Job drawing, mm, ordinate dimensions from the low corner. One solid piece. Give positions to 0.01 mm unless a question says otherwise; leave off trailing zeros. Order: outer loops, then holes, each group sorted by start corner. A loop starts at its lowest first (then second) coordinate and runs counter-clockwise, first axis right, second up. Notation, with made-up numbers: (-29.75, 52) -> (-10.75, 52) arc R10 cw to (-10.75, 58) -> close; hole circle Ø2 at (22.25, 22). An arc over 180 degrees is marked (long way). Use CSV: the item, a comma, the result in double quotes. Start each with the question number.
1. Cut at D-D on x = 15. List the corners of the cut face in (y, z).
2. Wall check: line 1 (Z direction, x = 1, y = 7.5); line 2 (Y direction, x = 2.1, z = 37); line 3 (Y direction, x = 12.75, z = 23). Give the ranges that are in metal, low to high. Write a range as from..to.
3. Cut at C-C on y = 33. List the corners of the cut face in (x, z).
4. Cut at A-A on x = 10. List the corners of the cut face in (y, z), then the cut area to 3 significant figures.
5. Cut at B-B on z = 32.5. List the corners of the cut face in (x, y), then the cut area to 3 significant figures.
6. Drop flat-ended pins along their axis: pin 1 (12 mm diameter, centred on x = 4, z = 36.5, fed in from -Y); pin 2 (5 mm diameter, centred on x = 2, z = 39, fed in from +Y); pin 3 (2 mm diameter, centred on y = 7.5, z = 37, fed in from -X). Give the stop position or say it passes through.
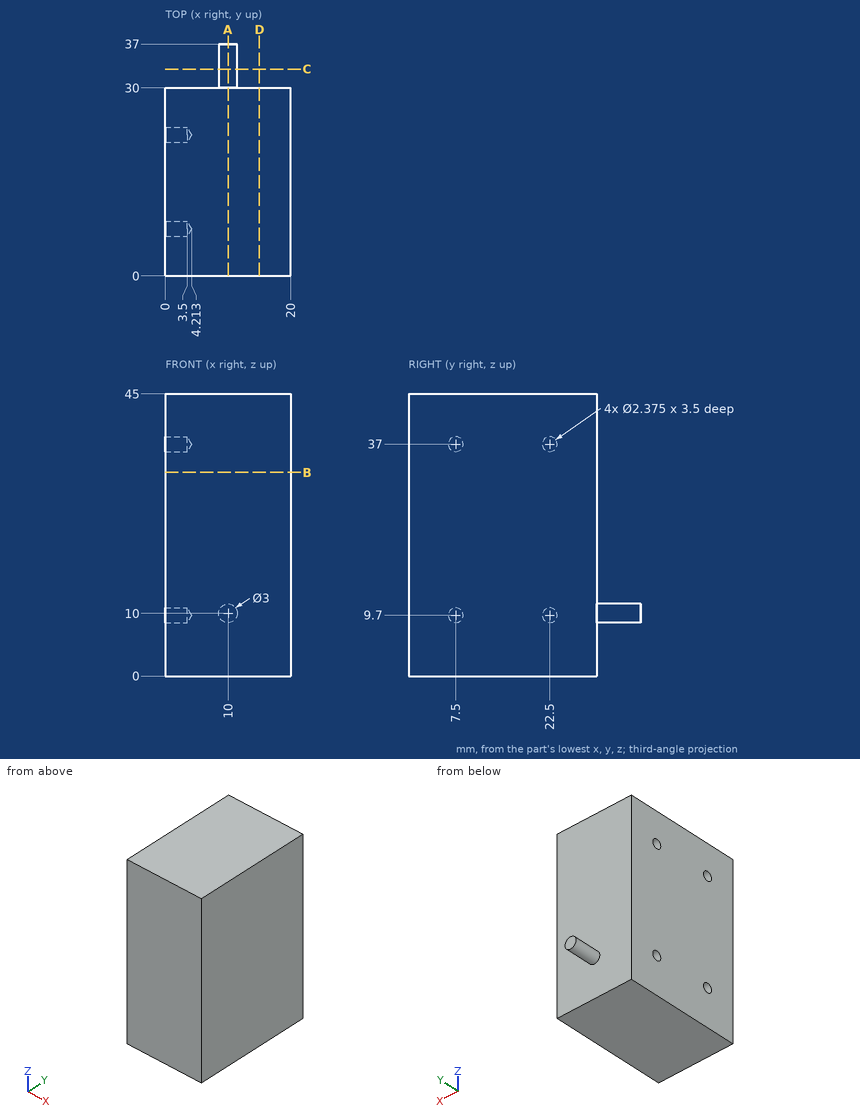
Verdict:
1,outline,"(0, 0) -> (30, 0) -> (30, 45) -> (0, 45) -> close"
2,line 1,"0..8.51, 10.89..35.81, 38.19..45"
2,line 2,"0..6.31, 8.69..21.31, 23.69..30"
2,line 3,"0..30"
3,outline,"circle Ø3 at (10, 10)"
4,outline,"(0, 0) -> (30, 0) -> (30, 8.5) -> (37, 8.5) -> (37, 11.5) -> (30, 11.5) -> (30, 45) -> (0, 45) -> close"
4,area,"1,370 mm^2"
5,outline,"(0, 0) -> (20, 0) -> (20, 30) -> (0, 30) -> close"
5,area,"600 mm^2"
6,pin 1,"y = 0"
6,pin 2,"y = 30"
6,pin 3,"x = 3.61"
